from build123d import *

# Parameters (mm, degrees)
SKETCH_2_W      = 98
SKETCH_2_H      = 98
EXTRUDE_1_DEPTH = 10
SKETCH_3_W      = 98
SKETCH_3_H      = 125
EXTRUDE_2_DEPTH = 10
SKETCH_4_W      = 98
SKETCH_4_H      = 62.5
EXTRUDE_3_DEPTH = 886.75
SKETCH_5_W      = 98
SKETCH_5_H      = 62.5
EXTRUDE_4_DEPTH = 7.1
SKETCH_6_W      = 98
SKETCH_6_H      = 62.5
EXTRUDE_5_DEPTH = 7.1
SKETCH_9_W      = 115.1
SKETCH_9_H      = 10
SKETCH_9_H_2    = 3.2
EXTRUDE_6_DEPTH = 102
SKETCH_11_W     = 50
SKETCH_11_H     = 1759.3
EXTRUDE_7_DEPTH = 62.5


with BuildPart() as part:
    # 草图2 → 凸台-拉伸1 (new body)
    with BuildSketch(Plane(origin=(0, 0, 0), x_dir=(1, 0, 0), z_dir=(0, 1, 0))):
        with Locations((34.507061985, 30.744472309)):
            Rectangle(SKETCH_2_W, SKETCH_2_H)
    extrude(amount=EXTRUDE_1_DEPTH)

    # 草图3 → 凸台-拉伸2 (add)
    with BuildSketch(Plane.XY.offset(18.255527691)):
        with Locations((34.507061985, -52.5)):
            Rectangle(SKETCH_3_W, SKETCH_3_H)
    extrude(amount=EXTRUDE_2_DEPTH)

    # 草图4 → 凸台-拉伸3 (add)
    with BuildSketch(Plane.XY.offset(28.255527691)):
        with Locations((34.507061985, -83.75)):
            Rectangle(SKETCH_4_W, SKETCH_4_H)
    extrude(amount=EXTRUDE_3_DEPTH)

    # 镜向4: part across plane


with BuildPart() as part_1:
    add(part.part)
    add(part.part.mirror(Plane.XY.offset(915.005527691)))

    # 草图5 → 凸台-拉伸4 (add)
    with BuildSketch(Plane.XY.offset(28.255527691)):
        with Locations((34.507061985, -21.25)):
            Rectangle(SKETCH_5_W, SKETCH_5_H)
    extrude(amount=EXTRUDE_4_DEPTH)

    # 草图6 → 凸台-拉伸5 (add)
    with BuildSketch(Plane(origin=(0, 0, 1801.755527691), x_dir=(-1, 0, 0), z_dir=(0, 0, -1))):
        with Locations((-34.507061985, -21.25)):
            Rectangle(SKETCH_6_W, SKETCH_6_H)
    extrude(amount=EXTRUDE_5_DEPTH)

    # 草图9 → 凸台-拉伸6 (add)
    with BuildSketch(Plane.ZY.offset(14.492938015)):
        with Locations((-22.194472309, 5)):
            Rectangle(SKETCH_9_W, SKETCH_9_H)
        with Locations((1852.205527691, 8.4)):
            Rectangle(SKETCH_9_W, SKETCH_9_H_2)
    extrude(amount=EXTRUDE_6_DEPTH)

    # 草图11 → 凸台-拉伸7 (add)
    with BuildSketch(Plane(origin=(0, -52.5, 0), x_dir=(1, 0, 0), z_dir=(0, 1, 0))):
        with Locations((58.507061985, -915.005527691)):
            Rectangle(SKETCH_11_W, SKETCH_11_H)
    extrude(amount=EXTRUDE_7_DEPTH)


solid = part_1.part
Part model, mm, in its own coordinate system. A direction names the side the tool comes from. Coordinates: 2 decimals unless noted, no trailing zeros. Loops run counter-clockwise (first coordinate to the right, second up) from the corner with the lowest first, then second, coordinate; pieces in that order, holes last. Notation, with made-up numbers: (19, -33.75) -> (30, -33.75) arc R21 cw to (30, -14.75) -> close; hole circle Ø6 at (36, 28). An arc over 180 degrees is marked (long way). Use a Markdown table: item, result. Add a question column.
Item 1: Which spindle directions (+Z, -Z, +X, -X, +Y, -Y) get a long thin tool onto all of the face, cutting with end or side? Do faces 5 (the flat face through (50, 10, 837)), 6 (the flat face through (-65, 6.8, 1851)), 7 (the flat face through (-7, -14, 1794.656)), 8 (the flat face through (34, -115, 928)), 9 (the flat face through (34, 0, 1861)). Say none if no direction does.
Item 2: Flat gauge pins, fed straight in: P1, Ø10, axis at y = -54, z = 935, coming from the -X side; P2, Ø14.5, axis at x = 19, z = 573.5, coming from the +Y side; P3, Ø10, axis at x = 49.5, y = -70.5, coming from the +Z side. Where does each tip first touch, or does it go through?
Item 3: Band-saw the part on D-D on y = -96. Write the cut outline in (x, z).
Item 4: Pull direction Z, two halves, no side cores. Call faces 1 (the flat face through (-7, -15, 35.356)), 2 (the flat face through (34, -57, 18.256)), 3 (the flat face through (9, -52.5, 927)), 4 (the flat face through (83.507, -53, 929)): +Z half, -Z half, draft (parallel to the pull), parting line (faces both ways), or undercut.
Item 5: Band-saw the part on B-B on z = 115. Write the cut outline in (x, y).
Item 6: Band-saw the part on C-C on x = 16.5. Write the cut outline in (y, z).
Item 7: Band-saw the part on A-A on x = -74. Write the cut outline in (y, z), plus the area to 3 significant figures.
Item 8: Probe probe 1 along Z at (x, y) = (-12, 4.5); probe 2 along X at (y, z) = (-108.5, 455.5); probe 3 along Z at (x, y) = (-8.5, -32). List the from-to ranges inside material, lowest first.
Geometry says:
| question | item | result |
|---|---|---|
| 1 | face 5 | +Z, -Z, +X, -X, +Y |
| 1 | face 6 | +Z, -X, -Y |
| 1 | face 7 | -X, +Y |
| 1 | face 8 | +Z, -Z, +X, -X, -Y |
| 1 | face 9 | +Z, +X, -X, -Y |
| 2 | P1 | x = -14.49 |
| 2 | P2 | y = -52.5 |
| 2 | P3 | z = 1811.76 |
| 3 | outline | (-14.49, 18.26) -> (83.51, 18.26) -> (83.51, 1811.76) -> (-14.49, 1811.76) -> close |
| 4 | face 1 | undercut |
| 4 | face 2 | -Z half |
| 4 | face 3 | undercut |
| 4 | face 4 | draft |
| 5 | outline | (-14.49, -115) -> (83.51, -115) -> (83.51, 10) -> (33.51, 10) -> (33.51, -52.5) -> (-14.49, -52.5) -> close |
| 6 | outline | (-115, 18.26) -> (0, 18.26) -> (0, -79.74) -> (10, -79.74) -> (10, 35.36) -> (-52.5, 35.36) -> (-52.5, 1794.66) -> (10, 1794.66) -> (10, 1909.76) -> (0, 1909.76) -> (0, 1811.76) -> (-115, 1811.76) -> close |
| 7 | outline | (0, -79.74) -> (10, -79.74) -> (10, 35.36) -> (0, 35.36) -> close; (6.8, 1794.66) -> (10, 1794.66) -> (10, 1909.76) -> (6.8, 1909.76) -> close |
| 7 | area | 1,520 mm² |
| 8 | probe 1 | -79.74 to 35.36, 1794.66 to 1909.76 |
| 8 | probe 2 | -14.49 to 83.51 |
| 8 | probe 3 | 18.26 to 35.36, 1794.66 to 1811.76 |
